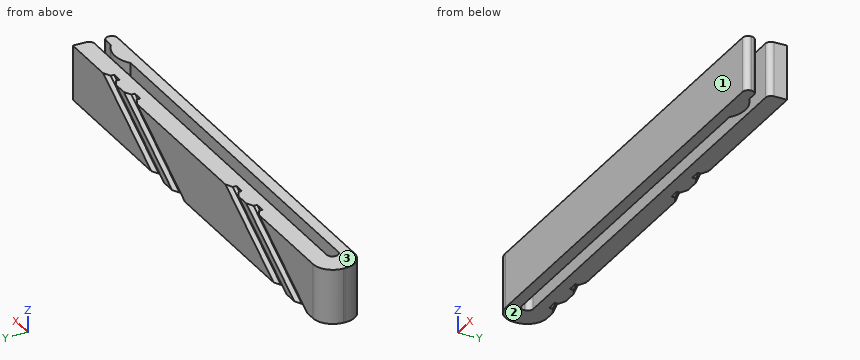
from build123d import *

# Parameters (mm, degrees)
F1_DEPTH    = 7.62
F3_DEPTH    = 1.016
F4_T1_DEPTH = 21.59
F5_R        = 0.762
F6_R        = 0.762
F7_SIZE     = 0.508


# Not quite as in the source:
# - a fillet or chamfer that OpenCascade refuses, or shapes differently, is made with other operations: its cross-section is extruded or revolved along the edge and cut away or added


with BuildPart() as f1:
    # F0 (on Top) → F1 (new body)
    with BuildSketch(Plane.XY):
        with BuildLine():
            Line((62.1792, 9.144), (-3.8608, 9.144))
            Line((-3.8608, 9.144), (-3.8608, 4.3472210688))
            Line((-3.8608, 4.3472210688), (62.1792, 4.3472210688))
            Line((62.1792, 4.3472210688), (62.1792, 5.9436))
            Line((62.1792, 5.9436), (60.087851236, 5.9436))
            ThreePointArc((60.087851236, 5.9436), (57.4883669615, 6.8209325844), (54.888882687, 5.9436))
            Line((54.888882687, 5.9436), (-0.5588, 5.9436))
            Line((-0.5588, 5.9436), (-0.5588, 7.5438))
            Line((-0.5588, 7.5438), (62.1792, 7.5438))
            Line((62.1792, 7.5438), (62.1792, 9.144))
        make_face()
    extrude(amount=F1_DEPTH)

    # F2 (on face) → F3 (join)
    with BuildSketch(Plane(origin=(0, 9.144, 0), x_dir=(-1, 0, 0), z_dir=(0, 1, 0))):
        Polygon((-14.0853170305, 7.62), (-1.3910392299, 0), (3.8608, 0), (3.8608, 7.62), align=None)
        Polygon((-19.5489563048, 7.62), (-6.8546785042, 0), (-2.8160745278, 0), (-15.5103523284, 7.62), align=None)
        Polygon((-33.6069809273, 0), (-8.279713802, 0), (-20.9739916027, 7.62), (-46.3012587279, 7.62), align=None)
        Polygon((-39.0706202015, 0), (-35.0320162252, 0), (-47.7262940258, 7.62), (-51.7648980021, 7.62), align=None)
        Polygon((-62.1792, 0), (-40.4956554994, 0), (-53.1899333, 7.62), (-62.1792, 7.62), align=None)
    extrude(amount=F3_DEPTH)

    # F4: fillet of radius 2.794 on 3 edges, made by hand

    # F4_s2 → F4_t1 (cut)
    with BuildSketch(Plane.XY.offset(-6.985)):
        with BuildLine():
            ThreePointArc((-1.0668, 4.3472210688), (-3.0424563466, 5.1655647222), (-3.8608, 7.1412210688))
            Line((-3.8608, 7.1412210688), (-3.8608, 4.3472210688))
            Line((-3.8608, 4.3472210688), (-1.0668, 4.3472210688))
        make_face()
        with BuildLine():
            ThreePointArc((-3.8608, 7.366), (-3.0424563466, 9.3416563466), (-1.0668, 10.16))
            Line((-1.0668, 10.16), (-3.8608, 10.16))
            Line((-3.8608, 10.16), (-3.8608, 7.366))
        make_face()
    extrude(amount=F4_T1_DEPTH, mode=Mode.SUBTRACT)

    # F5
    f5_edges = [f1.edges().sort_by_distance(p)[0] for p in [
        (-0.5588, 5.9436, 3.81),
        (-0.5588, 7.5438, 3.81),
    ]]
    fillet(f5_edges, radius=F5_R)

    # F6
    f6_edges = [f1.edges().sort_by_distance(p)[0] for p in [
        (62.1792, 7.5438, 3.81),
        (60.087851, 5.9436, 3.81),
        (62.1792, 5.9436, 3.81),
        (62.1792, 4.347221, 3.81),
    ]]
    fillet(f6_edges, radius=F6_R)

    # F7
    f7_edges = [f1.edges().sort_by_distance(p)[0] for p in [
        (7.738178, 10.16, 3.81),
        (9.163213, 10.16, 3.81),
        (13.201817, 10.16, 3.81),
        (14.626853, 10.16, 3.81),
        (39.95412, 10.16, 3.81),
        (41.379155, 10.16, 3.81),
        (45.417759, 10.16, 3.81),
        (46.842794, 10.16, 3.81),
    ]]
    chamfer(f7_edges, length=F7_SIZE)


solid = f1.part
Work out the finished part from the listing and answer in its coordinate system (mm). Face numbers are marked on the shaded views. Coordinates: 2 decimals unless noted, no trailing zeros. Loops run counter-clockwise (first coordinate to the right, second up) from the corner with the lowest first, then second, coordinate; pieces in that order, holes last. Notation, with made-up numbers: M 53,14 L 67,14 A25 ccw 67,32 Z; hole C -24.75,-29 d8. An arc over 180 degrees is marked long. Answer in a Markdown table with one row per item. Add a question column.
1. Consider L1, parallel to Y at x = 27, z = 6.5; L2, parallel to Y at x = 58, z = 6.5; L3, parallel to X at y = 9.3, z = 5. Determine where each line is inside the solid, lowest interval first.
2. Find section B-B, the plane x = 7.5. Write down the section's boundary in (y, z), then the cut area to 3 significant figures.
3. Find section D-D, the plane x = 57.5. Write down the section's boundary in (y, z), then the cut area to 3 significant figures.
4. A flat-ended cylindrical pin translates along its axis: P1, Ø1, axis at y = 9, z = 5.5, coming from the -X side. Find the tip coordinate at first contact, or state that the pin passes through.
5. Find section A-A, the plane x = 27. Write down the section's boundary in (y, z), then the cut area to 3 significant figures.
6. The mould has two halves that part along Z. Classify the marked faces 1, 2 and 3: pulls with the +Z half, pulls with the -Z half, needs draft (parallel to the pull), parting line crosses it, or undercut.
7. Find section C-C, the plane x = 18. Write down the section's boundary in (y, z), then the cut area to 3 significant figures.
Reported:
| question | item | result |
|---|---|---|
| 1 | L1 | y = 4.35 to 5.94, 7.54 to 10.16 |
| 1 | L2 | y = 4.35 to 6.79, 7.54 to 10.16 |
| 1 | L3 | x = -3.08 to 9.72, 11.15 to 15.18, 16.61 to 41.94, 43.36 to 47.4, 48.83 to 62.18 |
| 2 | outline | M 4.35,0 L 5.94,0 L 5.94,7.62 L 4.35,7.62 Z; M 7.54,0 L 9.14,0 L 9.14,0.39 L 9.65,0.39 L 10.16,0.98 L 10.16,2.22 L 9.65,2.81 L 9.14,2.81 L 9.14,3.67 L 9.65,3.67 L 10.16,4.26 L 10.16,7.62 L 7.54,7.62 Z |
| 2 | area | 30.4 mm^2 |
| 3 | outline | M 4.35,0 L 6.82,0 L 6.82,7.62 L 4.35,7.62 Z; M 7.54,0 L 10.16,0 L 10.16,7.62 L 7.54,7.62 Z |
| 3 | area | 38.8 mm^2 |
| 4 | P1 | stops at x = -3.62 |
| 5 | outline | M 4.35,0 L 5.94,0 L 5.94,7.62 L 4.35,7.62 Z; M 7.54,0 L 10.16,0 L 10.16,7.62 L 7.54,7.62 Z |
| 5 | area | 32.1 mm^2 |
| 6 | face 1 | needs draft |
| 6 | face 2 | pulls with the -Z half |
| 6 | face 3 | pulls with the +Z half |
| 7 | outline | M 4.35,0 L 5.94,0 L 5.94,7.62 L 4.35,7.62 Z; M 7.54,0 L 10.16,0 L 10.16,5.24 L 9.65,5.83 L 9.14,5.83 L 9.14,6.69 L 9.65,6.69 L 10.16,7.28 L 10.16,7.62 L 7.54,7.62 Z |
| 7 | area | 30.9 mm^2 |
